```python
from build123d import *

# Parameters (mm, degrees)
F0_W     = 48
F0_H     = 106
F1_DEPTH = 8
F2_W     = 24
F2_H     = 106
F3_DEPTH = 24
F4_R     = 6
F5_DEPTH = 40
F6_R     = 8


with BuildPart() as f1:
    # F0 (on Front) → F1 (new body)
    with BuildSketch(Plane.XZ):
        with Locations((-23.98444, 1.00732)):
            Rectangle(F0_W, F0_H)
    extrude(amount=F1_DEPTH)

    # F2 (on face) → F3 (join)
    with BuildSketch(Plane.XZ.offset(8)):
        with Locations((-11.98444, 1.00732)):
            Rectangle(F2_W, F2_H)
    extrude(amount=F3_DEPTH)

    # F4 (on face) → F5 (cut)
    with BuildSketch(Plane.XZ.offset(8)):
        with Locations((-35.98444, 42.00732)):
            Circle(F4_R)
        with Locations((-35.98444, -39.99268)):
            Circle(F4_R)
    extrude(amount=-F5_DEPTH, mode=Mode.SUBTRACT)

    # F6
    f6_edges = [f1.edges().sort_by_distance(p)[0] for p in [
        (-47.98444, -4, 54.00732),
        (-47.98444, -4, -51.99268),
    ]]
    fillet(f6_edges, radius=F6_R)


solid = f1.part
```
Part model, mm, in its own coordinate system. A direction names the side the tool comes from. Give positions to 0.01 mm unless a question says otherwise; leave off trailing zeros. Write each loop counter-clockwise with the first axis right and the second up, starting at its lowest first coordinate (ties: lowest second). Pieces come first, ordered by that corner, then holes. Notation, with made-up numbers: (-39.75, 74) -> (-29.75, 74) arc R23 ccw to (-29.75, 98) -> close; hole circle Ø8 at (1.5, -21). An arc over 180 degrees is marked (long way). Put each result on its own line as item: value. Start each with the question number.
Item 1: Cut at A-A (x = -33.5). List the corners of the cut face in (y, z), then the cut area to 3 significant figures.
Item 2: Cut at B-B (z = 44.5). List the corners of the cut face in (x, y), then the cut area to 3 significant figures.
Item 3: Which spindle directions (+Z, -Z, +X, -X, +Y, -Y) get a long thin tool onto all of the face, cutting with end or side? Do faces 1 (the face through (-16, -12, 54.007)), 2 (the face through (-23.984, -20, 0)). Say none if no direction does.
Item 4: Pin check, flat tips, straight feed: pin 1 Ø2 at (x, z) = (-19, 14.5) entering from +Y; pin 2 Ø8 at (y, z) = (-15, -23.5) entering from -X; pin 3 Ø7 at (x, z) = (-33.5, 10) entering from -Y. Stop position of each tip, or through.
Item 5: Wall check: L1, parallel to X at y = -13, z = -14.5; L2, parallel to Y at x = -24.5, z = 34.5. Give the ranges that are in metal, low to high. Write a range as [from, to].
Item 6: Cut at D-D (z = -2). List the corners of the cut face in (x, y).
Item 7: Pull direction Z, two halves, no side cores. Call faces 3 (the face through (-45.58, -4.06, -49.71)), 4 (the face through (-32.759, -4.056, -34.933)), 5 (the face through (-36, -8, 2)): pulls with the +Z half, pulls with the -Z half, needs draft (parallel to the pull), parting line crosses it, or undercut.
Item 8: Cut at C-C (y = -5.5). List the corners of the cut face in (x, z).
Answer list:
1. outline: (-8, -51.99) -> (0, -51.99) -> (0, -45.45) -> (-8, -45.45) -> close; (-8, -34.53) -> (0, -34.53) -> (0, 36.55) -> (-8, 36.55) -> close; (-8, 47.47) -> (0, 47.47) -> (0, 54.01) -> (-8, 54.01) -> close
1. area: 673 mm2
2. outline: (-47.98, -8) -> (-41.44, -8) -> (-41.44, 0) -> (-47.98, 0) -> close; (-30.53, -8) -> (-23.98, -8) -> (-23.98, -32) -> (0.02, -32) -> (0.02, 0) -> (-30.53, 0) -> close
2. area: 873 mm2
3. face 1: +Z, +X, -X, +Y, -Y
3. face 2: +Z, -Z, -X, -Y
4. pin 1: stops at y = 0
4. pin 2: stops at x = -23.98
4. pin 3: stops at y = -8
5. L1: x = [-23.98, 0.02]
5. L2: y = [-8, 0]
6. outline: (-47.98, -8) -> (-23.98, -8) -> (-23.98, -32) -> (0.02, -32) -> (0.02, 0) -> (-47.98, 0) -> close
7. face 3: pulls with the -Z half
7. face 4: undercut
7. face 5: needs draft
8. outline: (-47.98, -43.99) arc R8 ccw to (-39.98, -51.99) -> (0.02, -51.99) -> (0.02, 54.01) -> (-39.98, 54.01) arc R8 ccw to (-47.98, 46.01) -> close; hole circle Ø12 at (-35.98, -39.99); hole circle Ø12 at (-35.98, 42.01)
